Geometry: final body of the model. Coordinates: model frame, mm. Face numbers are marked on the shaded views. Give positions to 0.01 mm unless a question says otherwise; leave off trailing zeros. Order: outer loops, then holes, each group sorted by start corner. A loop starts at its lowest first (then second) coordinate and runs counter-clockwise, first axis right, second up. Notation, with made-up numbers: (75, -24) - (127, -24) arc R17 ccw to (127, 1) - close; hole circle Ø5 at (81, -33.75). An arc over 180 degrees is marked (long way). One line per item, written item: value.
Autodesk Inventor part; units mm, degrees
ref_plane "YZ Plane" through (0, 0, 0) normal (1, 0, 0) x (0, 1, 0)
ref_plane "XZ Plane" through (0, 0, 0) normal (0, 1, 0) x (-1, 0, 0)
ref_plane "XY Plane" through (0, 0, 0) normal (0, 0, 1) x (1, 0, 0)
sketch "Sketch1" plane through (0, 0, 0) normal (0, 0, 1) x (1, 0, 0)
  line L0 (-127, 0) -> (127, 0)
  line L1 (-127, -787.4) -> (-127, 0)
  line L2 (127, 0) -> (127, -787.4)
  line L3 (-63.5, -190.5) -> (63.5, -190.5) construction
  line L4 (63.5, -190.5) -> (63.5, -63.5) construction
  line L5 (63.5, -63.5) -> (-63.5, -63.5) construction
  line L6 (-63.5, -63.5) -> (-63.5, -190.5) construction
  line L7 (-63.5, -190.5) -> (63.5, -63.5) construction
  line L8 (63.5, -190.5) -> (-63.5, -63.5) construction
  circle A0 centre (-63.5, -63.5) radius 9.525
  circle A1 centre (63.5, -63.5) radius 9.525
  circle A2 centre (63.5, -190.5) radius 9.525
  circle A3 centre (-63.5, -190.5) radius 9.525
  line L9 (-127, -787.4) -> (127, -787.4)
  point P0 (0, 0)
  point P1 (0, 0)
  point P2 (0, -127)
  point P3 (0, -63.5)
  dimension "d1" = 254
  dimension "d7" = 19.05
  dimension "d8" = 127
  dimension "d9" = 127
  dimension "d10" = 63.5
extrude "Plate1" add sketch "Sketch1" along normal blind 9.525
sketch "Sketch3" plane through (-140.208, -787.4, 22.733) normal (-1, 0, 0) x (0, -1, 0)
  line L0 (-787.4, 0) -> (0, 0)
  line L1 (0, 0) -> (0, 37.592)
  line L2 (0, 37.592) -> (-787.4, 37.592)
  line L3 (-787.4, 37.592) -> (-787.4, 0)
edge flange "Flange2" height 50.8 angle 90 thickness 9.525 bend radius 13.208 thickness toward (-1, 0, 0) relief tear relief width 9.525 relief depth 4.7625 corner gap 9.525 corner form 0 edges at (-127, -393.7, 9.525) (127, -393.7, 9.525) wall of the first edge with corners at (-140.208, 0, 22.733) (-140.208, -787.4, 22.733) (-140.208, -787.4, 60.325) (-140.208, 0, 60.325)
bend "Bend2"
corner "Corner2"
sketch "Sketch4" plane through (0, 0, 0) normal (0, 0, -1) x (-1, 0, 0)
  line L0 (-38.1, -584.2) -> (38.1, -584.2)
  line L1 (50.8, -596.9) -> (50.8, -673.1)
  line L2 (38.1, -685.8) -> (-38.1, -685.8)
  line L3 (-50.8, -673.1) -> (-50.8, -596.9)
  line L4 (-50.8, -584.2) -> (50.8, -685.8) construction
  line L5 (50.8, -584.2) -> (-50.8, -685.8) construction
  line L6 (127, -787.4) -> (-127, -787.4)
  line L7 (-127, 0) -> (127, 0)
  arc A0 (-38.1, -584.2) -> (-50.8, -596.9) centre (-38.1, -596.9) ccw
  arc A1 (50.8, -596.9) -> (38.1, -584.2) centre (38.1, -596.9) ccw
  arc A2 (38.1, -685.8) -> (50.8, -673.1) centre (38.1, -673.1) ccw
  arc A3 (-50.8, -673.1) -> (-38.1, -685.8) centre (-38.1, -673.1) ccw
  point P0 (0, 0)
  point P1 (0, -635)
  point P2 (0, 0)
  dimension "d40" = 101.6
  dimension "d41" = 101.6
  dimension "d42" = 101.6
  dimension "d43" = 12.7
extrude "Cut1" cut sketch "Sketch4" against normal blind 9.525
equation "\"d44\" = Thickness"
equation "\"d15\" = Thickness"
equation "\"d30\" = BendReliefWidth"
equation "\"d31\" = BendReliefDepth"
equation "\"d32\" = MinimumRemnant"
equation "\"d33\" = TransitionRadius"
equation "\"d36\" = BendRadius"
equation "\"d37\" = CornerReliefSize"
equation "\"d38\" = GapSize"
equation "\"d39\" = JacobiRadiusSize"
equation "\"BendReliefWidth\" = Thickness"
equation "\"BendReliefDepth\" = 0.5 * Thickness"
equation "\"CornerReliefSize\" = 4 * Thickness"
equation "\"MinimumRemnant\" = 2 * Thickness"
equation "\"TransitionRadius\" = BendRadius"
equation "\"JacobiRadiusSize\" = Thickness"
equation "\"GapSize\" = Thickness"
properties part number "Model-5_Sheet-LH" material "SS304"
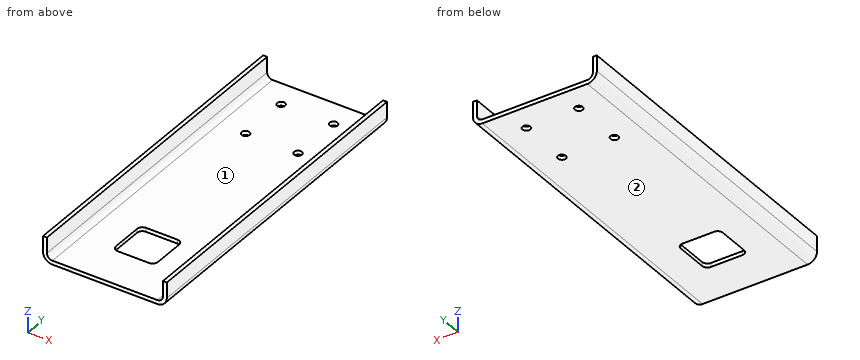
1) Section C-C, the plane z = 48. Return loops of the section in (x, y), then the cut area to 3 significant figures.
Answers below:
outline: (-149.73, -787.4) - (-140.21, -787.4) - (-140.21, 0) - (-149.73, 0) - close; (140.21, -787.4) - (149.73, -787.4) - (149.73, 0) - (140.21, 0) - close
area: 15,000 mm^2
2) First-contact query: pin 1 (10 mm diameter, centred on x = 2.5, y = -146.5, fed in from -Z); pin 2 (10.5 mm diameter, centred on y = -638.5, z = 5, fed in from -X); pin 3 (10 mm diameter, centred on x = -26, y = -132.5, fed in from +Z) (3 decimals); pin 4 (10.5 mm diameter, centred on y = -629.5, z = 2.5, fed in from +X). Flat tips, straight axial feed; report the tip coordinate or a pass-through.
Answers below:
pin 1: z = 0
pin 2: x = -146
pin 3: z = 9.525
pin 4: x = 144.1
3) Mould query, pull axis X, two halves, no side actions, for the marked faces 1 and 2. Classes: released by +X, released by -X, zero draft, split by the parting line, or undercut.
Answers below:
face 1: undercut
face 2: zero draft
4) Section D-D, the plane y = -651. Return loops of the section in (x, z) (3 decimals), then the cut area to 3 significant figures.
Answers below:
outline: (-149.733, 22.733) arc R22.733 ccw to (-127, 0) - (-50.8, 0) - (-50.8, 9.525) - (-127, 9.525) arc R13.208 cw to (-140.208, 22.733) - (-140.208, 60.325) - (-149.733, 60.325) - close; (50.8, 0) - (127, 0) arc R22.733 ccw to (149.733, 22.733) - (149.733, 60.325) - (140.208, 60.325) - (140.208, 22.733) arc R13.208 cw to (127, 9.525) - (50.8, 9.525) - close
area: 2,710 mm^2
5) Section B-B, the plane x = 63.5. Return loops of the section in (y, z) (3 decimals), then the cut area to 3 significant figures.
Answers below:
outline: (-787.4, 0) - (-200.025, 0) - (-200.025, 9.525) - (-787.4, 9.525) - close; (-180.975, 0) - (-73.025, 0) - (-73.025, 9.525) - (-180.975, 9.525) - close; (-53.975, 0) - (0, 0) - (0, 9.525) - (-53.975, 9.525) - close
area: 7,140 mm^2
6) Material intervals for line 1 along Y through (x, z) = (-63.5, 3.25) (3 decimals); line 2 along X through (y, z) = (-207.5, 48); line 3 along X through (y, z) = (-63, 4), sorted ascending.
Answers below:
line 1: -787.4 to -200.025, -180.975 to -73.025, -53.975 to 0
line 2: -149.73 to -140.21, 140.21 to 149.73
line 3: -139.88 to -73.01, -53.99 to 53.99, 73.01 to 139.88
7) Section A-A, the plane y = -63.5. Return loops of the section in (x, z) (3 decimals).
Answers below:
outline: (-149.733, 22.733) arc R22.733 ccw to (-127, 0) - (-73.025, 0) - (-73.025, 9.525) - (-127, 9.525) arc R13.208 cw to (-140.208, 22.733) - (-140.208, 60.325) - (-149.733, 60.325) - close; (-53.975, 0) - (53.975, 0) - (53.975, 9.525) - (-53.975, 9.525) - close; (73.025, 0) - (127, 0) arc R22.733 ccw to (149.733, 22.733) - (149.733, 60.325) - (140.208, 60.325) - (140.208, 22.733) arc R13.208 cw to (127, 9.525) - (73.025, 9.525) - close
